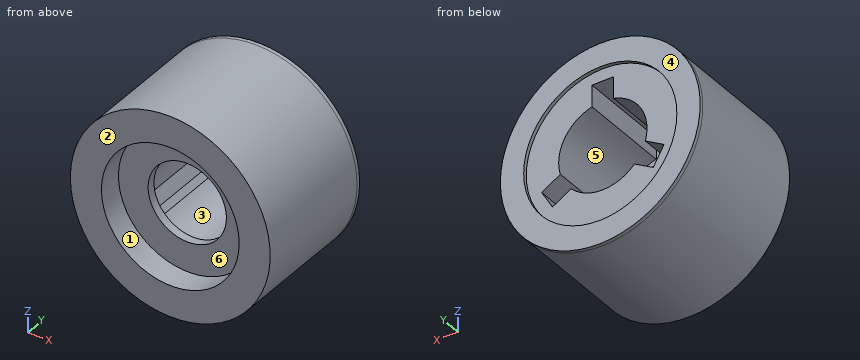
from build123d import *

# Parameters (mm, degrees)
F0_R      = 4.07
F1_DEPTH  = 5.111
F2_R      = 2.805
F3_DEPTH  = 1
F4_R      = 1.8
F5_DEPTH  = 3.77
F6_R      = 1.595
F7_DEPTH  = 4.112
F9_DEPTH  = 3.8
F10_R     = 4.07
F10_R_2   = 3.12
F11_DEPTH = 0.15


with BuildPart() as f1:
    # F0 (on Front) → F1 (new body)
    with BuildSketch(Plane.XZ):
        with Locations((-37.221067, 44.138376)):
            Circle(F0_R)
    extrude(amount=F1_DEPTH)

    # F2 (on face) → F3 (cut)
    with BuildSketch(Plane.XZ.offset(5.111)):
        with Locations((-37.221067, 44.138376)):
            Circle(F2_R)
    extrude(amount=-F3_DEPTH, mode=Mode.SUBTRACT)

    # F4 (on face) → F5 (cut)
    with BuildSketch(Plane(origin=(0, 0, 0), x_dir=(-1, 0, 0), z_dir=(0, 1, 0))):
        with Locations((37.221067, 44.138376)):
            Circle(F4_R)
    extrude(amount=-F5_DEPTH, mode=Mode.SUBTRACT)

    # F6 (on face) → F7 (cut, through all)
    with BuildSketch(Plane.XZ.offset(4.111)):
        with Locations((-37.221067, 44.138376)):
            Circle(F6_R)
    extrude(amount=-F7_DEPTH, mode=Mode.SUBTRACT)

    # F8 (on face) → F9 (cut)
    with BuildSketch(Plane(origin=(0, 0, 0), x_dir=(-1, 0, 0), z_dir=(0, 1, 0))):
        Polygon((36.780077, 46.764019), (36.780077, 45.88352), (37.660077, 45.884019), (37.660077, 46.764019), align=None)
        Polygon((34.727688, 43.205748), (35.167688, 42.443646), (35.930222, 42.883896), (35.48979, 43.645748), align=None)
        Polygon((39.275435, 42.44536), (39.715435, 43.207462), (38.952901, 43.647712), (38.513333, 42.88536), align=None)
    extrude(amount=-F9_DEPTH, mode=Mode.SUBTRACT)

    # F10 (on face) → F11 (join)
    with BuildSketch(Plane(origin=(0, 0, 0), x_dir=(-1, 0, 0), z_dir=(0, 1, 0))):
        with Locations((37.221067, 44.138376)):
            Circle(F10_R)
        with Locations((37.221067, 44.138376)):
            Circle(F10_R_2, mode=Mode.SUBTRACT)
    extrude(amount=F11_DEPTH)


solid = f1.part
Design review of the part built by this model. Coordinates are the model's own, in mm. Face numbers are marked on the shaded views. A direction names the side the tool comes from. Coordinates: 2 decimals unless noted, no trailing zeros. Loops run counter-clockwise (first coordinate to the right, second up) from the corner with the lowest first, then second, coordinate; pieces in that order, holes last. Notation, with made-up numbers: M 44,0.25 L 58,0.25 A20 cw 58,4.25 Z; hole C -35.75,67 d10. An arc over 180 degrees is marked long. Answer as CSV lines item,"result".
Item 1: The part is to be moulded in two halves that separate along Z. For the marked faces 4, 5 and 6, say which applies: pulls with the +Z half, pulls with the -Z half, needs draft (parallel to the pull), parting line crosses it, or undercut.
Answer list:
face 4,"needs draft"
face 5,"undercut"
face 6,"undercut"
Item 2: For probe 1 along Z at (x, y) = (-37.25, -1.65); probe 2 along X at (y, z) = (-4.2, 44.25); probe 3 along Z at (x, y) = (-37.75, -2), list the stretches that pass through material, from the lowest coordinate up.
Answer list:
probe 1,"40.07 to 42.34, 46.76 to 48.21"
probe 2,"-41.29 to -40.02, -34.42 to -33.15"
probe 3,"40.1 to 42.42, 45.86 to 48.17"
Item 3: Add section D-D on x = -39.5. State the section outline as (y, z) points, plus the area to 3 significant figures.
Answer list:
outline,"M -5.11,40.77 L 0.15,40.77 L 0.15,42.01 L 0,42.01 L 0,42.83 L -3.8,42.83 L -3.8,43.33 L 0,43.33 L 0,46.27 L 0.15,46.27 L 0.15,47.51 L -5.11,47.51 L -5.11,45.77 L -4.11,45.77 L -4.11,42.5 L -5.11,42.5 Z"
area,"29.7 mm²"
Item 4: Machinability: for the marked faces 1, 2 and 3, which of the approach directions +Z, -Z, +X, -X, +Y, -Y give a long, thin tool a straight path to every point of the face, cutting with its end or side? Answer none if there is none.
Answer list:
face 1,"-Y"
face 2,"+Z, -Z, +X, -X, -Y"
face 3,"+Y"
Item 5: For P1, Ø3, axis at y = -2.5, z = 45.5, coming from the +X side; P2, Ø1.5, axis at y = -3.5, z = 42.5, coming from the -X side; P3, Ø1, axis at x = -35.5, z = 43, coming from the +Y side; P4, Ø1, axis at y = -1, z = 46.5, coming from the +X side, all flat-tipped, find the tip position at first contact; note any pin that passes through.
Answer list:
P1,"x = -33.15"
P2,"x = -41.19"
P3,"y = 0"
P4,"x = -33.6"
Item 6: Add section B-B on z = 45. State the section outline as (x, y) points, plus the area to 3 significant figures.
Answer list:
outline,"M -41.2,-5.11 L -39.89,-5.11 L -39.89,-4.11 L -38.56,-4.11 L -38.56,-3.77 L -38.8,-3.77 L -38.8,0 L -40.22,0 L -40.22,0.15 L -41.2,0.15 Z; M -35.88,-4.11 L -34.55,-4.11 L -34.55,-5.11 L -33.24,-5.11 L -33.24,0.15 L -34.22,0.15 L -34.22,0 L -35.64,0 L -35.64,-3.77 L -35.88,-3.77 Z"
area,"22.8 mm²"
